Verification items for the finished model (mm, model axes). Face numbers are marked on the shaded views. A direction names the side the tool comes from. Coordinates: 2 decimals unless noted, no trailing zeros. Write each loop counter-clockwise with the first axis right and the second up, starting at its lowest first coordinate (ties: lowest second). Pieces come first, ordered by that corner, then holes. Notation, with made-up numbers: (-18, 30.25) -> (38, 30.25) arc R17 cw to (38, 50.25) -> close; hole circle Ø3 at (48, -38.75). An arc over 180 degrees is marked (long way). Answer in a Markdown table with one row per item.
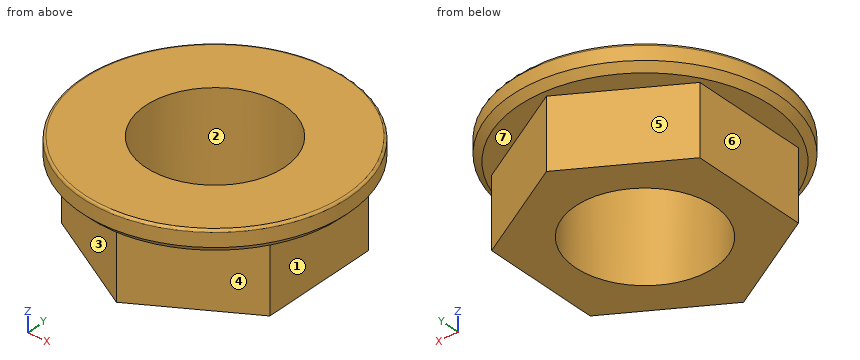
```python
from build123d import *

# Parameters (mm, degrees)
F0_R     = 3
F1_DEPTH = 3
F2_R     = 5.75
F2_R_2   = 3
F3_DEPTH = 1
F4_SIZE  = 0.3
F5_R     = 0.1


with BuildPart() as f1:
    # F0 (on Top) → F1 (new body)
    with BuildSketch(Plane.XY):
        Polygon((4.5, -2.598076), (4.5, 2.598076), (0, 5.196152), (-4.5, 2.598076), (-4.5, -2.598076), (0, -5.196152), align=None)
        Circle(F0_R, mode=Mode.SUBTRACT)
    extrude(amount=F1_DEPTH)

    # F2 (on face) → F3 (join)
    with BuildSketch(Plane.XY.offset(3)):
        Circle(F2_R)
        Circle(F2_R_2, mode=Mode.SUBTRACT)
    extrude(amount=F3_DEPTH)

    # F4
    f4_edges = [f1.edges().sort_by_distance(p)[0] for p in [
        (-5.75, 0, 3),
    ]]
    chamfer(f4_edges, length=F4_SIZE)

    # F5
    f5_edges = [f1.edges().sort_by_distance(p)[0] for p in [
        (-5.75, 0, 4),
    ]]
    fillet(f5_edges, radius=F5_R)


solid = f1.part
```
1. Mould release check, pull along Y, two halves, no side actions. Record for the marked faces 1, 2 and 3: released by +Y, released by -Y, zero draft, split by the parting line, or undercut.
Geometry says:
| item | result |
|---|---|
| face 1 | zero draft |
| face 2 | undercut |
| face 3 | released by -Y |
2. Tool access check on the marked faces 4, 5, 6 and 7. Record the directions out of +Z, -Z, +X, -X, +Y, -Y that give a thin tool (end or side, any length) a straight path to the whole face; none if there is none.
Geometry says:
| item | result |
|---|---|
| face 4 | -Z, +X, -Y |
| face 5 | -Z, -X, +Y |
| face 6 | -Z, -X, +Y, -Y |
| face 7 | -Z |
3. Section check B-B, the plane z = 0.95. Record the boundary of the cut face in (x, y).
Geometry says:
| item | result |
|---|---|
| outline | (-4.5, -2.6) -> (0, -5.2) -> (4.5, -2.6) -> (4.5, 2.6) -> (0, 5.2) -> (-4.5, 2.6) -> close; hole circle Ø6 at (0, 0) |
4. Depth check by flat-ended pin: P1, Ø0.9, axis at y = -1, z = 1, coming from the +X side; P2, Ø1.5, axis at y = -1, z = 2, coming from the -X side; P3, Ø1.5, axis at y = -3, z = 2.5, coming from the -X side. Enter the tip coordinate at first touch or a pass-through.
Geometry says:
| item | result |
|---|---|
| P1 | x = 4.5 |
| P2 | x = -4.5 |
| P3 | x = -4.95 |
5. Section check A-A, the plane y = 0. Record the boundary of the cut face in (x, z).
Geometry says:
| item | result |
|---|---|
| outline | (-5.75, 3.3) -> (-5.45, 3) -> (-4.5, 3) -> (-4.5, 0) -> (-3, 0) -> (-3, 4) -> (-5.65, 4) arc R0.1 ccw to (-5.75, 3.9) -> close; (3, 0) -> (4.5, 0) -> (4.5, 3) -> (5.45, 3) -> (5.75, 3.3) -> (5.75, 3.9) arc R0.1 ccw to (5.65, 4) -> (3, 4) -> close |
6. Thickness scan on line 1 (Z direction, x = 0.5, y = 5); line 2 (X direction, y = 0.25, z = 0.8); line 3 (Y direction, x = -3.5, z = 3.25). Record the ranges inside material, lowest first. Write a range as from..to.
Geometry says:
| item | result |
|---|---|
| line 1 | 3..4 |
| line 2 | -4.5..-2.99, 2.99..4.5 |
| line 3 | -4.5..4.5 |
